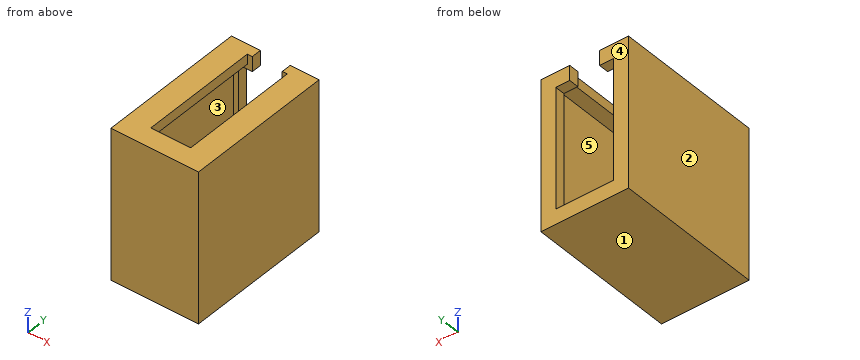
Autodesk Inventor part; units mm, degrees
ref_plane "YZ Plane" through (0, 0, 0) normal (1, 0, 0) x (0, 1, 0)
ref_plane "XZ Plane" through (0, 0, 0) normal (0, 1, 0) x (-1, 0, 0)
ref_plane "XY Plane" through (0, 0, 0) normal (0, 0, 1) x (1, 0, 0)
sketch "Sketch1" plane through (0, 0, 0) normal (0, 1, 0) x (-1, 0, 0)
  line L0 (-3.4, 6.55) -> (3.4, 6.55)
  line L1 (3.4, 6.55) -> (3.4, -6.55)
  line L2 (3.4, -6.55) -> (-3.4, -6.55)
  line L3 (-3.4, -6.55) -> (-3.4, 6.55)
  line L4 (-3.4, 6.55) -> (3.4, -6.55) construction
  line L5 (3.4, 6.55) -> (-3.4, -6.55) construction
  line L6 (4.4, -7.55) -> (4.4, 7.55)
  line L7 (4.4, 7.55) -> (-4.4, 7.55)
  line L8 (-4.4, 7.55) -> (-4.4, -7.55)
  line L9 (-4.4, -7.55) -> (4.4, -7.55)
  point P0 (0, 0)
  dimension "d0" = 6.8
  dimension "d1" = 13.1
  dimension "d2" = 1
extrude "Extrusion1" add sketch "Sketch1" along normal blind 14
sketch "Sketch3" plane through (0, 0, 0) normal (0, -1, 0) x (1, 0, 0)
  line L0 (-4.4, 7.55) -> (4.4, 7.55)
  line L1 (-4.4, -7.55) -> (-4.4, 7.55)
  line L2 (4.4, -7.55) -> (-4.4, -7.55)
  line L3 (4.4, 7.55) -> (4.4, -7.55)
  line L4 (-3.4, -6.55) -> (3.4, -6.55)
  line L5 (-3.4, 6.55) -> (-3.4, -6.55)
  line L6 (3.4, 6.55) -> (-3.4, 6.55)
  line L7 (3.4, -6.55) -> (3.4, 6.55)
  point P0 (0, 0)
extrude "Extrusion2" add sketch "Sketch3" along normal blind 1 contours L0 L3 L2 L1 | L5 L6 L7 L4
sketch "Sketch4" plane through (-4.4, 14, 7.55) normal (0, 0, 1) x (1, 0, 0)
  line L0 (0, 0) -> (8.8, 0)
  line L1 (2.4, 0) -> (6.4, 0)
  line L2 (6.4, 0) -> (6.4, -13)
  line L3 (6.4, -13) -> (2.4, -13)
  line L4 (2.4, -13) -> (2.4, 0)
  point P0 (4.4, -14)
  point P1 (4.4, 0)
  point P2 (4.4, 0)
  point P3 (6.4, 0)
  dimension "d7" = 1
  dimension "d8" = 4
extrude "Extrusion3" cut sketch "Sketch4" against normal up to surface (1 mm away)
sketch "Sketch5" plane through (0, 14, 0) normal (0, 1, 0) x (1, 0, 0)
  line L0 (2, -6.55) -> (2, -7.55)
  line L1 (2, -7.55) -> (4.4, -7.55)
  line L2 (4.4, -7.55) -> (4.4, 7.55)
  line L3 (4.4, 7.55) -> (-4.4, 7.55)
  line L4 (-4.4, 7.55) -> (-4.4, -7.55)
  line L5 (-4.4, -7.55) -> (-2, -7.55)
  line L6 (-2, -7.55) -> (-2, -6.55)
  line L7 (-2, -6.55) -> (-3.4, -6.55)
  line L8 (-3.4, -6.55) -> (-3.4, 6.55)
  line L9 (-3.4, 6.55) -> (3.4, 6.55)
  line L10 (3.4, 6.55) -> (3.4, -6.55)
  line L11 (3.4, -6.55) -> (2, -6.55)
  line L12 (-2.9, 6.05) -> (-2.9, -6.05)
  line L13 (-2.9, -6.05) -> (-1.5, -6.05)
  line L14 (-1.5, -6.05) -> (-1.5, -8.05)
  line L15 (-1.5, -8.05) -> (-4.9, -8.05)
  line L16 (-4.9, -8.05) -> (-4.9, 8.05)
  line L17 (-4.9, 8.05) -> (4.9, 8.05)
  line L18 (4.9, 8.05) -> (4.9, -8.05)
  line L19 (4.9, -8.05) -> (1.5, -8.05)
  line L20 (1.5, -8.05) -> (1.5, -6.05)
  line L21 (1.5, -6.05) -> (2.9, -6.05)
  line L22 (2.9, -6.05) -> (2.9, 6.05)
  line L23 (2.9, 6.05) -> (-2.9, 6.05)
  line L24 (-4.4, -7.55) -> (-2, -7.55)
  line L25 (-2, -7.55) -> (-1.5, -7.55)
  line L26 (4.4, -7.55) -> (-4.4, -7.55)
  line L27 (2, -7.55) -> (2, -6.55)
  line L28 (2, -7.55) -> (1.5, -7.55)
  point P0 (0, 0)
  point P1 (1.5, -7.55)
  dimension "d11" = 0.5
extrude "Extrusion4" add sketch "Sketch5" against normal blind 1 contours L0 L26 L20 L21 L22 L23 L12 L13 L14 L25 L6 L7 L8 L9 L10 L11
properties part number "SwitchHolder" material "Thermoplastic Resin"
For this review, take the finished solid that the model builds, in its own axes (mm). Face numbers are marked on the shaded views. A direction names the side the tool comes from. Coordinates: 2 decimals unless noted, no trailing zeros. Order: outer loops, then holes, each group sorted by start corner. A loop starts at its lowest first (then second) coordinate and runs counter-clockwise, first axis right, second up. Notation, with made-up numbers: (65, 79) - (104, 79) arc R24 ccw to (104, 115) - close; hole circle Ø10 at (5, 22.25). An arc over 180 degrees is marked (long way). Answer as a JSON object with one key per item and string values. Group by question number.
1. We need section B-B on y = 0.25. State the section outline as (x, z) points, then the cut area to 3 significant figures.
2. The part is to be moulded in two halves that separate along Z. For the marked faces 1, 2 and 3, say which applies: pulls with the +Z half, pulls with the -Z half, needs draft (parallel to the pull), parting line crosses it, or undercut.
3. We need section D-D on y = 13.25. State the section outline as (x, z) points.
4. For probe 1 along X at (y, z) = (5, -2.5); probe 2 along Z at (x, y) = (3, 4.75); probe 3 along Y at (x, z) = (-3, -1.25), list the stretches that pass through material, from the lowest coordinate up.
5. We need section A-A on z = -6.25. State the section outline as (x, y) points.
6. We need section C-C on x = -0.5. State the section outline as (y, z) points, then the cut area to 3 significant figures.
7. Clearance check with flat-ended pins moving along their axes: P1, Ø3.5, axis at x = -0.5, y = 8.5, coming from the +Z side; P2, Ø1.1, axis at x = -0.5, y = 13.5, coming from the +Z side. State where each tip first meets the part, or that it passes through.
8. For the marked faces 4 and 5, list the 3-axis set-ups (+Z, -Z, +X, -X, +Y, -Y) from which the entire face can be reached by the end or side of a thin tool; tool diameter is ignored.
Final values:
{
 "1": {"outline": "(-4.4, -7.55) - (4.4, -7.55) - (4.4, 7.55) - (-4.4, 7.55) - close; hole (-3.4, -6.55) - (3.4, -6.55) - (3.4, 6.55) - (-3.4, 6.55) - close", "area": "43.8 mm²"},
 "2": {"face 1": "pulls with the -Z half", "face 2": "needs draft", "face 3": "undercut"},
 "3": {"outline": "(-4.4, -7.55) - (4.4, -7.55) - (4.4, 7.55) - (1.5, 7.55) - (1.5, 6.05) - (2.9, 6.05) - (2.9, -6.05) - (-2.9, -6.05) - (-2.9, 6.05) - (-1.5, 6.05) - (-1.5, 7.55) - (-4.4, 7.55) - close"},
 "4": {"probe 1": "-4.4 to -3.4, 3.4 to 4.4", "probe 2": "-7.55 to -6.55, 6.55 to 7.55", "probe 3": "-1 to 0, 13 to 14"},
 "5": {"outline": "(-4.4, -1) - (4.4, -1) - (4.4, 14) - (-4.4, 14) - close; hole (-3.4, 0) - (3.4, 0) - (3.4, 13) - (-3.4, 13) - close"},
 "6": {"outline": "(-1, -7.55) - (14, -7.55) - (14, -6.05) - (13, -6.05) - (13, -6.55) - (0, -6.55) - (0, 6.55) - (1, 6.55) - (1, 7.55) - (-1, 7.55) - close", "area": "30.6 mm²"},
 "7": {"P1": "z = 7.55", "P2": "z = -6.05"},
 "8": {"face 4": "+Z, -Z, +X, -X, +Y", "face 5": "none"}
}
